Geometry: final body of the model. Coordinates: model frame, mm. Face numbers are marked on the shaded views. A direction names the side the tool comes from. Coordinates: 2 decimals unless noted, no trailing zeros. Write each loop counter-clockwise with the first axis right and the second up, starting at its lowest first coordinate (ties: lowest second). Pieces come first, ordered by that corner, then holes.
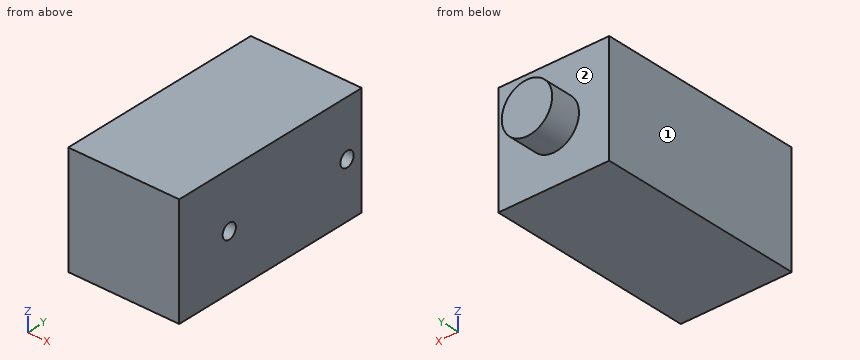
from build123d import *

# Parameters (mm, degrees)
SKETCH1_W           = 33
SKETCH1_H           = 33
BOSS_EXTRUDE1_DEPTH = 62
SKETCH2_R           = 7.5
BOSS_EXTRUDE2_DEPTH = 9.1
SKETCH3_R           = 2.25
CUT_EXTRUDE1_DEPTH  = 9.1


with BuildPart() as part:
    # Sketch1 → Boss-Extrude1 (new body)
    with BuildSketch(Plane(origin=(0, 0, 0), x_dir=(1, 0, 0), z_dir=(0, 1, 0))):
        Rectangle(SKETCH1_W, SKETCH1_H)
    extrude(amount=BOSS_EXTRUDE1_DEPTH)

    # Sketch2 → Boss-Extrude2 (add)
    with BuildSketch(Plane(origin=(0, 62, 0), x_dir=(1, 0, 0), z_dir=(0, 1, 0))):
        with Locations(Location((0, 0, 0), (0, 0, 270))):
            Circle(SKETCH2_R)
    extrude(amount=BOSS_EXTRUDE2_DEPTH)

    # Sketch3 → Cut-Extrude1 (cut)
    with BuildSketch(Plane(origin=(16.5, 0, 0), x_dir=(0, 0, -1), z_dir=(1, 0, 0))):
        with Locations((0, 57)):
            Circle(SKETCH3_R)
        with Locations((0, 17)):
            Circle(SKETCH3_R)
    extrude(amount=-CUT_EXTRUDE1_DEPTH, mode=Mode.SUBTRACT)


solid = part.part
Item 1: Section D-D, the plane z = 1.5. Output: boundary loops of the cut face in (x, y), plus the area to 3 significant figures.
Derived:
outline: (-16.5, 0) - (16.5, 0) - (16.5, 15.32) - (7.4, 15.32) - (7.4, 18.68) - (16.5, 18.68) - (16.5, 55.32) - (7.4, 55.32) - (7.4, 58.68) - (16.5, 58.68) - (16.5, 62) - (7.35, 62) - (7.35, 71.1) - (-7.35, 71.1) - (-7.35, 62) - (-16.5, 62) - close
area: 2,120 mm2
Item 2: Set-up query: the marked faces 1 and 2. Return all of +Z, -Z, +X, -X, +Y, -Y with unobstructed straight access to the full face (end or side cutting, diameter ignored); none if empty.
Derived:
face 1: +Z, -Z, -X, +Y, -Y
face 2: +Y
Item 3: Section B-B, the plane x = 14.5. Output: boundary loops of the cut face in (y, z), plus the area to 3 significant figures.
Derived:
outline: (0, -16.5) - (62, -16.5) - (62, 16.5) - (0, 16.5) - close; hole circle Ø4.5 at (17, 0); hole circle Ø4.5 at (57, 0)
area: 2,010 mm2
Item 4: Section C-C, the plane x = 0. Output: boundary loops of the cut face in (y, z), plus the area to 3 significant figures.
Derived:
outline: (0, -16.5) - (62, -16.5) - (62, -7.5) - (71.1, -7.5) - (71.1, 7.5) - (62, 7.5) - (62, 16.5) - (0, 16.5) - close
area: 2,180 mm2
Item 5: Material intervals for probe 1 along Y at (x, z) = (12, 0); probe 2 along Y at (x, z) = (12, -1); probe 3 along Y at (x, z) = (7.5, -5), sorted ascending.
Derived:
probe 1: y = 0 to 14.75, 19.25 to 54.75, 59.25 to 62
probe 2: y = 0 to 14.98, 19.02 to 54.98, 59.02 to 62
probe 3: y = 0 to 62
Item 6: Pin query (flat end, axial travel): pin 1 (2 mm diameter, centred on x = 1.5, z = 12, fed in from +Y). Return the tip coordinate at first contact, or that it passes through.
Derived:
pin 1: stops at y = 62
Item 7: Section A-A, the plane y = 17. Output: boundary loops of the cut face in (x, z), plus the area to 3 significant figures.
Derived:
outline: (-16.5, -16.5) - (16.5, -16.5) - (16.5, -2.25) - (7.4, -2.25) - (7.4, 2.25) - (16.5, 2.25) - (16.5, 16.5) - (-16.5, 16.5) - close
area: 1,050 mm2
